Input: part model. Units: mm. Frame: model coordinates. Give positions to 0.01 mm unless a question says otherwise; leave off trailing zeros. Order: outer loops, then holes, each group sorted by start corner. A loop starts at its lowest first (then second) coordinate and runs counter-clockwise, first axis right, second up. Notation, with made-up numbers: M 60,65.25 L 115,65.25 A27 ccw 115,100.25 Z; hole C 89,-8 d11. An arc over 180 degrees is marked long. Use a Markdown table: item, result.
from build123d import *

# Parameters (mm, degrees)
F0_R          = 10
F1_DEPTH      = 25
F2_DEPTH      = 25
F2_DEPTH_BACK = 25
F3_SIZE       = 2


with BuildPart() as f1:
    # F0 (on Front) → F1 (new body)
    with BuildSketch(Plane.XZ):
        with BuildLine():
            ThreePointArc((2.083333, -24.913043), (18.399502, -16.92508), (25, 0))
            ThreePointArc((25, 0), (18.399502, 16.92508), (2.083333, 24.913043))
            ThreePointArc((2.083333, 24.913043), (-25, 0), (2.083333, -24.913043))
        make_face()
        Circle(F0_R, mode=Mode.SUBTRACT)
        with BuildLine():
            ThreePointArc((2.083333, 24.913043), (18.399502, 16.92508), (25, 0))
            ThreePointArc((25, 0), (18.399502, -16.92508), (2.083333, -24.913043))
            Line((2.083333, -24.913043), (91.458333, -17.43913))
            ThreePointArc((91.458333, -17.43913), (72.5, 0), (91.458333, 17.43913))
            Line((91.458333, 17.43913), (2.083333, 24.913043))
        make_face()
        with BuildLine():
            ThreePointArc((107.5, 0), (102.879651, 11.847556), (91.458333, 17.43913))
            ThreePointArc((91.458333, 17.43913), (72.5, 0), (91.458333, -17.43913))
            ThreePointArc((91.458333, -17.43913), (102.879651, -11.847556), (107.5, 0))
        make_face()
        with Locations((90, 0)):
            Circle(F0_R, mode=Mode.SUBTRACT)
    extrude(amount=F1_DEPTH)

    # F0 (on Front) → F2 (join, two sides)
    with BuildSketch(Plane.XZ) as f2_sk:
        with BuildLine():
            ThreePointArc((2.083333, -24.913043), (18.399502, -16.92508), (25, 0))
            ThreePointArc((25, 0), (18.399502, 16.92508), (2.083333, 24.913043))
            ThreePointArc((2.083333, 24.913043), (-25, 0), (2.083333, -24.913043))
        make_face()
        Circle(F0_R, mode=Mode.SUBTRACT)
    extrude(amount=F2_DEPTH)
    extrude(f2_sk.sketch, amount=-F2_DEPTH_BACK)

    # F3
    f3_edges = [f1.edges().sort_by_distance(p)[0] for p in [
        (80, 0, 0),
        (-2.083333, 25, 24.913043),
        (-10, 25, 0),
    ]]
    chamfer(f3_edges, length=F3_SIZE)


solid = f1.part
1) Cut plane C-C on x = 90. Return loops of the section in (y, z).
Response values:
| item | result |
|---|---|
| outline | M -25,-17.56 L 0,-17.56 L 0,-12 L -2,-10 L -25,-10 Z; M -25,10 L -2,10 L 0,12 L 0,17.56 L -25,17.56 Z |
2) Material intervals for line 1 (Z direction, x = 0, y = -6); line 2 (Y direction, x = 53, z = 14.5); line 3 (Z direction, x = -4, y = -4.5), sorted ascending. Write a range as from..to.
Response values:
| item | result |
|---|---|
| line 1 | z = -25..-10, 10..25 |
| line 2 | y = -25..0 |
| line 3 | z = -24.68..-9.17, 9.17..24.68 |
3) Cut plane B-B on y = -7.5. Return loops of the section in (x, z), and give its area (3 significant figures).
Response values:
| item | result |
|---|---|
| outline | M 2.08,-24.91 L 91.46,-17.44 A17.5 ccw 91.46,17.44 L 2.08,24.91 A25 ccw long Z; hole C 0,0 d20; hole C 90,0 d20 |
| area | 4,670 mm² |
4) Mould query, pull axis Z, two halves, no side actions, for faces 1 (the face through (47.396, -12.325, 21.124)), 2 (the face through (-2.17, -0.66, -9.76)), 3 (the face through (46.15, -12.32, -21.23)). Classes: released by +Z, released by -Z, zero draft, split by the parting line, or undercut.
Response values:
| item | result |
|---|---|
| face 1 | released by +Z |
| face 2 | undercut |
| face 3 | released by -Z |
5) Cut plane A-A on x = 0. Return loops of the section in (y, z), and give its area (3 significant figures).
Response values:
| item | result |
|---|---|
| outline | M -25,-25 L 23,-25 L 25,-23 L 25,-12 L 23,-10 L -25,-10 Z; M -25,10 L 23,10 L 25,12 L 25,23 L 23,25 L -25,25 Z |
| area | 1,490 mm² |
6) Cut plane D-D on z = -8.5. State how many separate pieces and enclosed holes the cut face has, and give its area (3 significant figures).
Response values:
| item | result |
|---|---|
| separate pieces | 3 |
| enclosed holes | 0 |
| area | 3,590 mm² |
7) First-contact query: pin 1 Ø3 at (y, z) = (-15.5, -14.5) entering from -X; pin 2 Ø1 at (x, y) = (-1.5, 6.5) entering from -Z; pin 3 Ø12 at (y, z) = (-19.5, 15.5) entering from -X. Flat tips, straight axial feed; report the tip coordinate or a pass-through.
Response values:
| item | result |
|---|---|
| pin 1 | stops at x = -21.35 |
| pin 2 | stops at z = -24.98 |
| pin 3 | stops at x = -23.12 |
